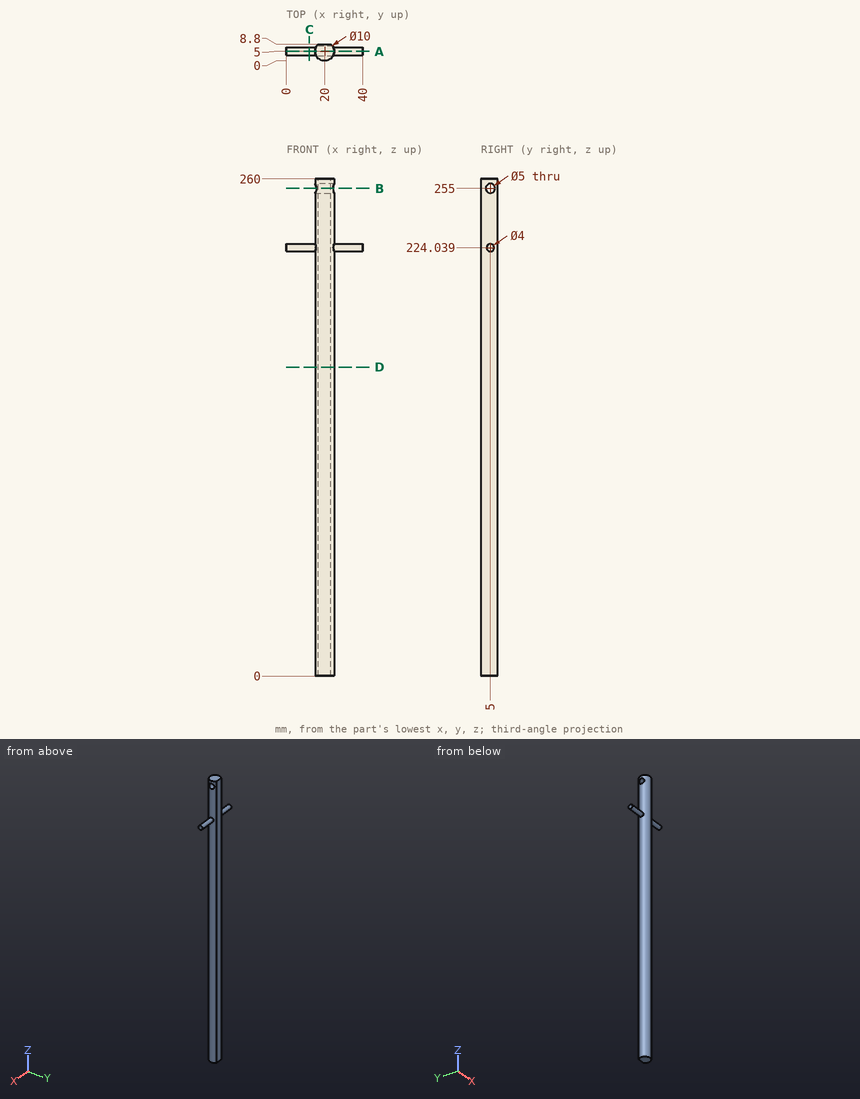
Input: dimensioned drawing with shaded views. Units: mm. Origin: part minimum x, y, z. Give positions to 0.01 mm unless a question says otherwise; leave off trailing zeros. Write each loop counter-clockwise with the first axis right and the second up, starting at its lowest first coordinate (ties: lowest second). Pieces come first, ordered by that corner, then holes.
Q1. First-contact query: P1, Ø4, axis at y = 5.5, z = 55, coming from the +X side; P2, Ø1.5, axis at x = 31, y = 5, coming from the -Z side; P3, Ø12, axis at x = 27.5, z = 87, coming from the -Y side. Flat tips, straight axial feed; report the tip coordinate or a pass-through.
Q2. Section B-B, the plane z = 255. Output: boundary loops of the cut face in (x, y).
Q3. Material intervals for probe 1 along Y at (x, z) = (21, 255); probe 2 along Y at (x, z) = (18, 255); probe 3 along X at (y, z) = (4.75, 26), sorted ascending.
Q4. Section C-C, the plane x = 12. Output: boundary loops of the cut face in (y, z).
Q5. Section A-A, the plane y = 5. Output: boundary loops of the cut face in (x, z), plus the area to 3 significant figures.
Q6. Section D-D, the plane z = 161.5. Output: boundary loops of the cut face in (x, y), plus the area to 3 significant figures.
Filled in:
1. P1: stops at x = 25
1. P2: stops at z = 222.04
1. P3: stops at y = 0.23
2. outline: (15.67, 2.5) arc R5 ccw to (24.33, 2.5) - close; (15.67, 7.5) - (24.33, 7.5) arc R5 ccw to (23.25, 8.8) - (16.75, 8.8) arc R5 ccw to start
3. probe 1: y = 0.1 to 2.5, 7.5 to 8.8
3. probe 2: y = 0.42 to 2.5, 7.5 to 8.8
3. probe 3: x = 15.01 to 24.99
4. outline: circle Ø4 at (5, 224.04)
5. outline: (0, 222.04) - (15, 222.04) - (15, 0) - (25, 0) - (25, 222.04) - (40, 222.04) - (40, 226.04) - (25, 226.04) - (25, 252.5) - (15, 252.5) - (15, 226.04) - (0, 226.04) - close; (15, 257.5) - (25, 257.5) - (25, 260) - (15, 260) - close
5. area: 2,670 mm2
6. outline: (16.75, 8.8) arc R5 ccw (long way) to (23.25, 8.8) - close
6. area: 73.2 mm2
